from build123d import *

# Parameters (mm, degrees)
CUT_EXTRUDE_2_DEPTH = 1.2
FILLET_1_R          = 0.1


with BuildPart() as part:
    # 草图8 → Revolve 1380 (revolve)
    with BuildSketch(Plane(origin=(0, 0, 0), x_dir=(0, 0, -1), z_dir=(1, 0, 0))):
        with BuildLine():
            Line((0, 0), (-15.4, 0))
            ThreePointArc((-15.4, 0), (-15.180811394, 1.464186604), (-14.542463035, 2.8))
            Line((-14.542463035, 2.8), (-13, 2.8))
            Line((-13, 2.8), (-13, 1.45))
            Line((-13, 1.45), (-2.511473671, 1.45))
            Line((-2.511473671, 1.45), (0, 0))
        make_face()
    revolve(axis=Axis((0, 0, 11.71), (0, 0, -1)))

    # 草图7 → 切除-拉伸2 (cut)
    with BuildSketch(Plane.XY.offset(15.4)):
        with BuildLine():
            Line((0.2, 0.928708781), (0.2, 0.797500009))
            ThreePointArc((0.2, 0.797500009), (0.375003701, 0.375003701), (0.797500009, 0.2))
            Line((0.797500009, 0.2), (0.928708781, 0.2))
            ThreePointArc((0.928708781, 0.2), (0.95, 0), (0.928708781, -0.2))
            Line((0.928708781, -0.2), (0.797500009, -0.2))
            ThreePointArc((0.797500009, -0.2), (0.375003701, -0.375003701), (0.2, -0.797500009))
            Line((0.2, -0.797500009), (0.2, -0.928708781))
            ThreePointArc((0.2, -0.928708781), (0, -0.95), (-0.2, -0.928708781))
            Line((-0.2, -0.928708781), (-0.2, -0.797500009))
            ThreePointArc((-0.2, -0.797500009), (-0.375003701, -0.375003701), (-0.797500009, -0.2))
            Line((-0.797500009, -0.2), (-0.928708781, -0.2))
            ThreePointArc((-0.928708781, -0.2), (-0.95, 0), (-0.928708781, 0.2))
            Line((-0.928708781, 0.2), (-0.797500009, 0.2))
            ThreePointArc((-0.797500009, 0.2), (-0.375003701, 0.375003701), (-0.2, 0.797500009))
            Line((-0.2, 0.797500009), (-0.2, 0.928708781))
            ThreePointArc((-0.2, 0.928708781), (0, 0.95), (0.2, 0.928708781))
        make_face()
    extrude(amount=-CUT_EXTRUDE_2_DEPTH, mode=Mode.SUBTRACT)

    # 圆角1
    fillet_1_edges = [part.edges().sort_by_distance(p)[0] for p in [
        (0, -1.45, 13),
    ]]
    fillet(fillet_1_edges, radius=FILLET_1_R)


solid = part.part
The listing builds one solid part. Answer for the finished solid, in the listing's coordinates (mm). A direction names the side the tool comes from. Coordinates: 2 decimals unless noted, no trailing zeros. Write each loop counter-clockwise with the first axis right and the second up, starting at its lowest first coordinate (ties: lowest second). Pieces come first, ordered by that corner, then holes. Notation, with made-up numbers: M 7,61 L 43,61 A19 ccw 43,84 Z; hole C -25,7 d8. An arc over 180 degrees is marked long. Use one line per item in the form item = value.
Item 1: Find section B-B, the plane y = 1.75. Give the vertices of the cut face in (x, z).
Model answer:
outline = M -2.19,13 L 2.19,13 L 2.19,14.54 A4.68 ccw -2.19,14.54 Z
Item 2: Find section C-C, the plane x = -2.2. Give the vertices of the cut face in (y, z), plus the area to 3 significant figures.
Model answer:
outline = M -1.73,13 L 1.73,13 L 1.73,14.54 A4.49 ccw -1.73,14.54 Z
area = 6.15 mm2
Item 3: For faces 4 (the face through (0.06, -1.45, 7.63)), 5 (the face through (0.1, -2.8, 13.8)), determine the directions among +Z, -Z, +X, -X, +Y, -Y from which every point of the face is accessible in a straight line to the end or side of a thin tool.
Model answer:
face_4 = -Z
face_5 = +Z, -Z
Item 4: Given P1, Ø2, axis at x = -2, z = 6, coming from the +Y side; P2, Ø1.5, axis at x = -0.5, z = 11.5, coming from the -Y side; P3, Ø1, axis at x = -1, y = -1.5, coming from the +Z side, each flat-ended and moving along its own axis, determine where each tip first touches the part or whether it passes through.
Model answer:
P1 = 1.05
P2 = -1.45
P3 = 15.23
Item 5: Find section D-D, the plane z = 4.75. Give the vertices of the cut face in (x, y).
Model answer:
outline = C 0,0 d2.9
Item 6: The mould has two halves that part along Y. Classify faces 1 (the face through (-1.21, 1.21, 13)), 2 (the face through (-0.34, -0.44, 0.96)), 3 (the face through (0, 0, 14.2)): released by +Y, released by -Y, zero draft, split by the parting line, or undercut.
Model answer:
face_1 = zero draft
face_2 = split by the parting line
face_3 = undercut
Item 7: Find the intervals of material crossed by probe 1 along Y at (x, z) = (-0.1, 9.5); probe 2 along Z at (x, y) = (-1.05, -0.2); probe 3 along Y at (x, z) = (-2.5, 14.5), in increasing order.
Model answer:
probe_1 = -1.45 to 1.45
probe_2 = 1.85 to 15.28
probe_3 = -1.26 to 1.26
Item 8: Find section A-A, the plane z = 13.5. Give the vertices of the cut face in (x, y), plus the area to 3 significant figures.
Model answer:
outline = C 0,0 d5.6
area = 24.6 mm2
